The model under review builds one solid part; all positions refer to its coordinate system, in mm. Coordinates: 2 decimals unless noted, no trailing zeros. Write each loop counter-clockwise with the first axis right and the second up, starting at its lowest first coordinate (ties: lowest second). Pieces come first, ordered by that corner, then holes. Notation, with made-up numbers: M 44.25,-10.5 L 63.25,-10.5 A26 ccw 63.25,27.5 Z; hole C -27,66.25 d8. An arc over 180 degrees is marked long. Answer as a JSON object with one key per item and string values.
Autodesk Inventor part; units mm, degrees
ref_plane "YZ Plane" through (0, 0, 0) normal (1, 0, 0) x (0, 1, 0)
ref_plane "XZ Plane" through (0, 0, 0) normal (0, 1, 0) x (-1, 0, 0)
ref_plane "XY Plane" through (0, 0, 0) normal (0, 0, 1) x (1, 0, 0)
sketch "Szkic1" plane through (0, 0, 0) normal (0, 0, 1) x (1, 0, 0)
  line L0 (0, 0) -> (115, 0) construction
  line L1 (0, -10) -> (115, -10)
  line L2 (115, 10) -> (0, 10)
  arc A0 (0, 10) -> (0, -10) centre (0, 0) ccw
  arc A1 (115, -10) -> (115, 10) centre (115, 0) ccw
  point P0 (57.5, 0)
  point P1 (40, 0)
  dimension "d0" = 115
  dimension "d1" = 20
  dimension "d2" = 75
extrude "Wyciągnięcie proste1" add sketch "Szkic1" along normal blind 3
hole "Otwór1" at (115, 0, 0) at (40, 0, 0) direction (0, 0, 1) diameter 6 end through all
hole "Otwór2" at (0, 0, 0) direction (0, 0, 1) diameter 6 end through all
properties part number "lacznik_zewn"
(1) Add section A-A on x = 40. Give the boundary of the cut face in (y, z).
Results list:
{"outline": "M -10,0 L -3,0 L -3,3 L -10,3 Z; M 3,0 L 10,0 L 10,3 L 3,3 Z"}
(2) Add section D-D on y = -5. Give the boundary of the cut face in (x, z), and give its area (3 significant figures).
Results list:
{"outline": "M -8.66,0 L 123.66,0 L 123.66,3 L -8.66,3 Z", "area": "397 mm²"}
(3) Wall thickness on line 1 along X through (y, z) = (0, 1.7); line 2 along Y through (x, z) = (0, 1); line 3 along X through (y, z) = (-2.5, 1.25): over which ranges is each line inside the solid? List them lowest first. Write a range as from..to.
Results list:
{"line 1": "-10..-3, 3..37, 43..112, 118..125", "line 2": "-10..-3, 3..10", "line 3": "-9.68..-1.66, 1.66..38.34, 41.66..113.34, 116.66..124.68"}
(4) For pin 1 Ø3.5 at (x, y) = (40, 0) entering from +Z; pin 2 Ø1.5 at (y, z) = (2.5, 2) entering from -X, all flat-tipped, find the tip position at first contact; note any pin that passes through.
Results list:
{"pin 1": "through", "pin 2": "x = -9.85"}
(5) Add section B-B on y = 0. Give the boundary of the cut face in (x, z).
Results list:
{"outline": "M -10,0 L -3,0 L -3,3 L -10,3 Z; M 3,0 L 37,0 L 37,3 L 3,3 Z; M 43,0 L 112,0 L 112,3 L 43,3 Z; M 118,0 L 125,0 L 125,3 L 118,3 Z"}
(6) Draft analysis for pull direction X (two halves, no side actions). For faces 1 (the face through (125, 0, 1)), 2 (the face through (58, 10, 1)), 3 (the face through (0, -3, 2)), state which applies: released by +X, released by -X, zero draft, split by the parting line, or undercut.
Results list:
{"face 1": "released by +X", "face 2": "zero draft", "face 3": "undercut"}
(7) Add section C-C on z = 1.6. Give the boundary of the cut face in (x, y).
Results list:
{"outline": "M 0,-10 L 115,-10 A10 ccw 115,10 L 0,10 A10 ccw Z; hole C 0,0 d6; hole C 40,0 d6; hole C 115,0 d6"}
